Here's how the part is built. I have some questions about the finished solid (model axes, mm). Face numbers are marked on the shaded views. A direction names the side the tool comes from. Round coordinates to 2 decimals unless told otherwise and drop trailing zeros. Loops run counter-clockwise (first coordinate to the right, second up) from the corner with the lowest first, then second, coordinate; pieces in that order, holes last. Notation, with made-up numbers: (38, 36.5) -> (94, 36.5) arc R27 ccw to (94, 71.5) -> close; hole circle Ø3 at (-2.75, -15). An arc over 180 degrees is marked (long way). Use CSV: the item, a comma, the result in double quotes. Start each with the question number.
from build123d import *

# Parameters (mm, degrees)
BOSS_EXTRUDE1_DEPTH     = 8.9
SKETCH4_W               = 94.9
SKETCH4_H               = 4.080124435
CUT_EXTRUDE1_DEPTH      = 77.015080741
CUT_EXTRUDE1_DEPTH_BACK = 77.015080741
SKETCH7_W               = 76.9
SKETCH7_H               = 2.319875565
CUT_EXTRUDE2_DEPTH      = 77.015080741
CUT_EXTRUDE2_DEPTH_BACK = 77.015080741
SKETCH8_R               = 3
CUT_EXTRUDE3_DEPTH      = 7.4
CUT_EXTRUDE3_DEPTH_BACK = 3.5


with BuildPart() as part:
    # Sketch3 → Boss-Extrude1 (new body)
    with BuildSketch(Plane(origin=(0, 0, 0), x_dir=(1, 0, 0), z_dir=(0, 1, 0))):
        with BuildLine():
            Line((-57.3, 49.95), (57.3, 49.95))
            ThreePointArc((57.3, 49.95), (76.015080741, 0), (57.3, -49.95))
            Line((57.3, -49.95), (-57.3, -49.95))
            ThreePointArc((-57.3, -49.95), (-76.015080741, 0), (-57.3, 49.95))
        make_face()
    extrude(amount=BOSS_EXTRUDE1_DEPTH)

    # Sketch4 → Cut-Extrude1 (cut, two sides)
    with BuildSketch(Plane(origin=(0, 0, 0), x_dir=(0, 0, -1), z_dir=(1, 0, 0))) as cut_extrude1_sk:
        with Locations((0, 4.540062218)):
            Rectangle(SKETCH4_W, SKETCH4_H)
    extrude(amount=CUT_EXTRUDE1_DEPTH, mode=Mode.SUBTRACT)
    extrude(cut_extrude1_sk.sketch, amount=-CUT_EXTRUDE1_DEPTH_BACK, mode=Mode.SUBTRACT)

    # Sketch7 → Cut-Extrude2 (cut, two sides)
    with BuildSketch(Plane(origin=(0, 0, 0), x_dir=(0, 0, -1), z_dir=(1, 0, 0))) as cut_extrude2_sk:
        with Locations((0, 7.740062218)):
            Rectangle(SKETCH7_W, SKETCH7_H)
    extrude(amount=CUT_EXTRUDE2_DEPTH, mode=Mode.SUBTRACT)
    extrude(cut_extrude2_sk.sketch, amount=-CUT_EXTRUDE2_DEPTH_BACK, mode=Mode.SUBTRACT)

    # Sketch8 → Cut-Extrude3 (cut, two sides)
    with BuildSketch(Plane(origin=(0, 2.5, 0), x_dir=(1, 0, 0), z_dir=(0, 1, 0))) as cut_extrude3_sk:
        Circle(SKETCH8_R)
    extrude(amount=CUT_EXTRUDE3_DEPTH, mode=Mode.SUBTRACT)
    extrude(cut_extrude3_sk.sketch, amount=-CUT_EXTRUDE3_DEPTH_BACK, mode=Mode.SUBTRACT)


solid = part.part
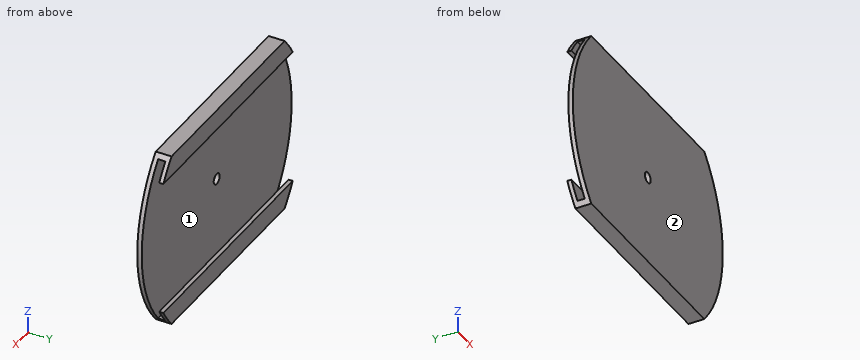
Q1. I want a section at D-D, the plane x = -18. List the corners of the cut face in (y, z) for me, then the cut area to 3 significant figures.
Q2. I want a section at C-C, the plane z = 0. List the corners of the cut face in (x, y) for me.
Q3. I want a section at B-B, the plane x = 0. List the corners of the cut face in (y, z) for me.
Q4. Will these pins go through, and if not, where does the flat tip stop? pin 1 Ø6 at (x, z) = (17, 31.5) entering from +Y; pin 2 Ø5 at (x, z) = (0, 0) entering from +Y.
Q5. I need wall thicknesses on line 1 along Z through (x, y) = (0, 1.4); line 2 along X through (y, z) = (1.5, 0); line 3 along Z through (x, y) = (0.5, 7.5). Which ranges of each line are inside material? Lowest first, please.
Q6. I want a section at A-A, the plane y = 4.25. List the corners of the cut face in (x, z) for me.
Q7. For the marked faces 1 and 2, which set-ups out of +Z, -Z, +X, -X, +Y, -Y let a thin tool reach every point of the face, with its end or its side?
Values found:
1,outline,"(0, -49.95) -> (8.9, -49.95) -> (8.9, -38.45) -> (6.58, -38.45) -> (6.58, -47.45) -> (2.5, -47.45) -> (2.5, 47.45) -> (6.58, 47.45) -> (6.58, 38.45) -> (8.9, 38.45) -> (8.9, 49.95) -> (0, 49.95) -> close"
1,area,"324 mm2"
2,outline,"(-76.02, 0) -> (-3, 0) -> (-3, 2.5) -> (-76.02, 2.5) -> close; (3, 0) -> (76.02, 0) -> (76.02, 2.5) -> (3, 2.5) -> close"
3,outline,"(0, -49.95) -> (8.9, -49.95) -> (8.9, -38.45) -> (6.58, -38.45) -> (6.58, -47.45) -> (2.5, -47.45) -> (2.5, -3) -> (0, -3) -> close; (0, 3) -> (2.5, 3) -> (2.5, 47.45) -> (6.58, 47.45) -> (6.58, 38.45) -> (8.9, 38.45) -> (8.9, 49.95) -> (0, 49.95) -> close"
4,pin 1,"y = 2.5"
4,pin 2,"through"
5,line 1,"-49.95 to -3, 3 to 49.95"
5,line 2,"-76.02 to -3, 3 to 76.02"
5,line 3,"-49.95 to -38.45, 38.45 to 49.95"
6,outline,"(-59.39, -47.45) arc R76.02 ccw to (-57.3, -49.95) -> (57.3, -49.95) arc R76.02 ccw to (59.39, -47.45) -> close; (-59.39, 47.45) -> (59.39, 47.45) arc R76.02 ccw to (57.3, 49.95) -> (-57.3, 49.95) arc R76.02 ccw to start"
7,face 1,"+X, -X"
7,face 2,"+Z, -Z, +X, -X, -Y"
